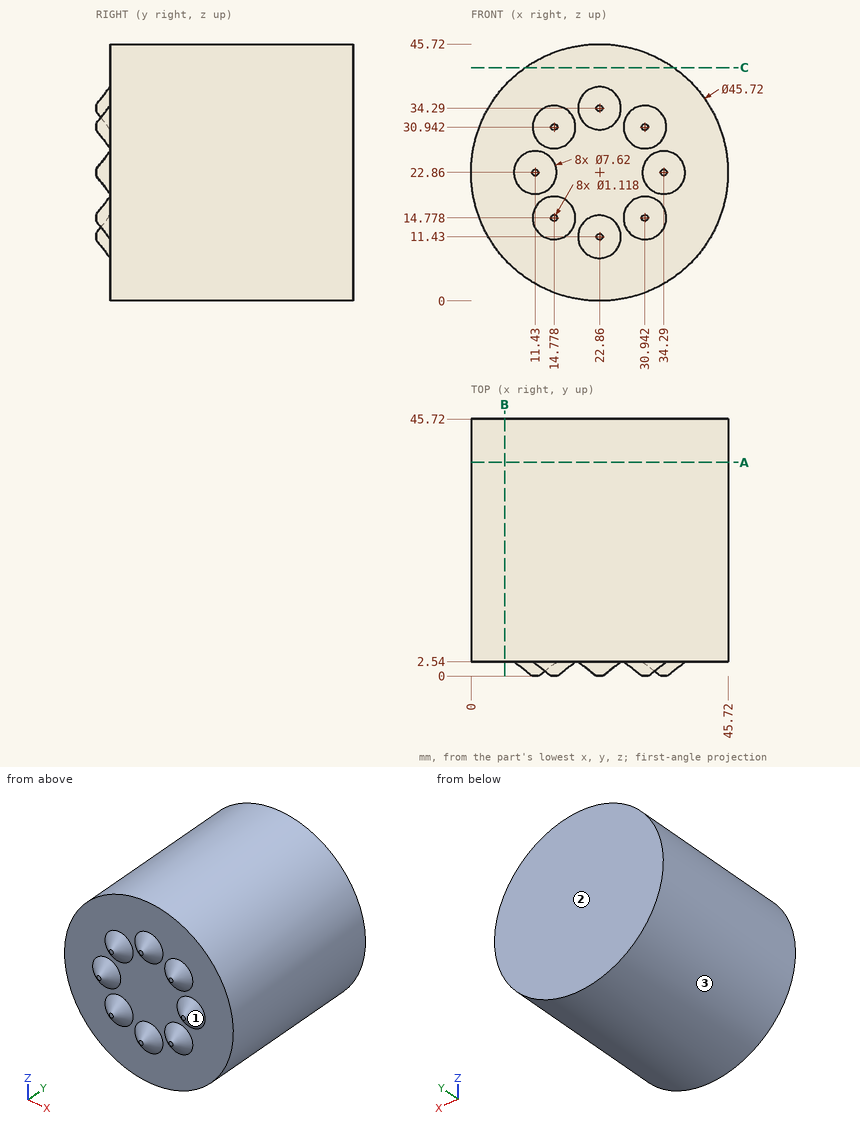
Verification items for this drawing (mm, ordinates from the low corner). Round coordinates to 2 decimals unless told otherwise and drop trailing zeros. Loops run counter-clockwise (first coordinate to the right, second up) from the corner with the lowest first, then second, coordinate; pieces in that order, holes last. Notation, with made-up numbers: (10.5, -14.5) - (15.5, -14.5) arc R23 ccw to (15.5, 12.5) - close; hole circle Ø1 at (29.5, -37.5). An arc over 180 degrees is marked (long way). Answer as CSV lines item,"result". Start each with the question number.
Item 1: Scan lines: line 1 (Z direction, x = 23.5, y = 19.5); line 2 (Y direction, x = 21.5, z = 16); line 3 (Z direction, x = 34, y = 15). Record each from-to range of solid material in increasing order. Write a range as [from, to].
Item 2: Section check A-A (y = 38). Record the boundary of the cut face in (x, z).
Item 3: Depth check by flat-ended pin: P1, Ø5, axis at y = 39.5, z = 30, coming from the +X side; P2, Ø4, axis at x = 31.5, z = 33, coming from the -Y side; P3, Ø10, axis at x = 37.5, y = 34, coming from the +Z side; P4, Ø10, axis at y = 24.5, z = 25.5, coming from the -X side. Enter the tip coordinate at first touch or a pass-through.
Item 4: Section check C-C (z = 41.5). Record the boundary of the cut face in (x, y).
Item 5: Section check B-B (x = 6). Record the boundary of the cut face in (y, z).
Item 6: Release check for a two-part mould opening along X. For the marked faces 1, 2 and 3 record: +X half, -X half, draft (parallel to the pull), parting line (faces both ways), or undercut.
Report:
1,line 1,"z = [0.01, 45.71]"
1,line 2,"y = [2.54, 45.72]"
1,line 3,"z = [2.9, 42.82]"
2,outline,"circle Ø45.72 at (22.86, 22.86)"
3,P1,"stops at x = 45.24"
3,P2,"stops at y = 0"
3,P3,"stops at z = 43.59"
3,P4,"stops at x = 0"
4,outline,"(9.63, 2.54) - (36.09, 2.54) - (36.09, 45.72) - (9.63, 45.72) - close"
5,outline,"(2.54, 7.42) - (45.72, 7.42) - (45.72, 38.3) - (2.54, 38.3) - close"
6,face 1,"undercut"
6,face 2,"draft"
6,face 3,"parting line"
